from build123d import *

# Parameters (mm, degrees)
SKETCH1_W                        = 60
SKETCH1_H                        = 65
BOSS_EXTRUDE2_DEPTH              = 3
BOSS_EXTRUDE4_DEPTH              = 150
CUT_EXTRUDE2_DEPTH               = 150
FILLET1_R                        = 10
SHELL1_T                         = -5
M10X1_25_TAPPED_HOLE1_AT_2_COUNT = 2
M10X1_25_TAPPED_HOLE1_AT_2_PITCH = 42.5


with BuildPart() as part:
    # Sketch1 → Boss-Extrude2 (new body)
    with BuildSketch(Plane(origin=(0, 0, 0), x_dir=(1, 0, 0), z_dir=(0, 1, 0))):
        with Locations((30, 32.5)):
            Rectangle(SKETCH1_W, SKETCH1_H)
    extrude(amount=BOSS_EXTRUDE2_DEPTH)

    # Sketch3 → Boss-Extrude4 (add)
    with BuildSketch(Plane(origin=(0, 3, 0), x_dir=(1, 0, 0), z_dir=(0, 1, 0))):
        Polygon((0, 0), (60, 0), (33.5, 60.392887062), (26.5, 60.392887062), align=None)
    extrude(amount=BOSS_EXTRUDE4_DEPTH)

    # Sketch5 → Cut-Extrude2 (cut)
    with BuildSketch(Plane.ZY):
        Polygon((-60.392887062, 3), (-5.391813619, 150.489864796), (0, 153), (0, 157.732510012), (-60.392887062, 157.732510012), align=None)
    extrude(amount=-CUT_EXTRUDE2_DEPTH, mode=Mode.SUBTRACT)

    # Fillet1
    fillet1_edges = [part.edges().sort_by_distance(p)[0] for p in [
        (0, 1.5, -65),
        (60, 1.5, -65),
    ]]
    fillet(fillet1_edges, radius=FILLET1_R)

    # Shell1
    shell1_openings = [part.faces().sort_by_distance(p)[0] for p in [
        (30, 52, 0),
    ]]
    offset(amount=SHELL1_T, openings=shell1_openings)

    # Sketch7 → M10x1.25 Tapped Hole1 (revolve, cut)
    with BuildSketch(Plane(origin=(51.25, 3, -43.980915379), x_dir=(0, 0, 1), z_dir=(1, 0, 0))):
        Polygon((0, 0), (0, 3), (4.4, 3), (4.4, 0.625), (5.025, 0), align=None)
    m10x1_25_tapped_hole1 = revolve(axis=Axis((51.25, 9.35, -43.980915379), (0, -1, 0)), mode=Mode.SUBTRACT)

    # M10x1.25 Tapped Hole1 at 2: M10x1.25 Tapped Hole1 ×2
    with Locations(*[(-i * M10X1_25_TAPPED_HOLE1_AT_2_PITCH, 0, 0) for i in range(1, M10X1_25_TAPPED_HOLE1_AT_2_COUNT)]):
        add(m10x1_25_tapped_hole1, mode=Mode.SUBTRACT)


solid = part.part
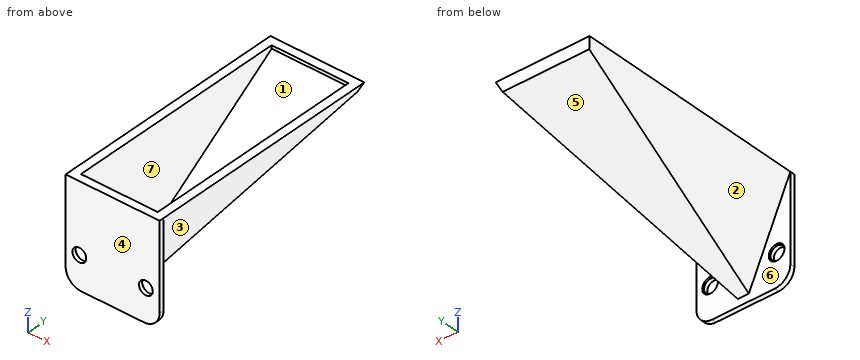
Check sheet for the modelled part. Datum: model origin and axes. Units: mm. Face numbers are marked on the shaded views. A direction names the side the tool comes from. Give positions to 0.01 mm unless a question says otherwise; leave off trailing zeros. Order: outer loops, then holes, each group sorted by start corner. A loop starts at its lowest first (then second) coordinate and runs counter-clockwise, first axis right, second up. Notation, with made-up numbers: (78.5, 25.25) - (137.5, 25.25) arc R32 ccw to (137.5, 59.25) - close; hole circle Ø9 at (56.25, 47). An arc over 180 degrees is marked (long way). Answer as CSV lines item,"result".
1. Section check A-A (z = -13). Record the boundary of the cut face in (x, y).
Result sheet:
outline,"(0, 0) - (60, 0) - (60, 3) - (54.3, 3) - (54.3, 130.09) - (5.7, 130.09) - (5.7, 3) - (0, 3) - close; hole (11.16, 5) - (48.84, 5) - (48.84, 115.78) - (11.16, 115.78) - close"
2. Mould release check, pull along X, two halves, no side actions. Record for the marked faces 1, 2, 3 and 4: released by +X, released by -X, zero draft, split by the parting line, or undercut.
Result sheet:
face 1,"undercut"
face 2,"released by -X"
face 3,"released by +X"
face 4,"zero draft"
3. Tool access check on the marked faces 5, 6 and 7. Record the directions out of +Z, -Z, +X, -X, +Y, -Y that give a thin tool (end or side, any length) a straight path to the whole face; none if there is none.
Result sheet:
face 5,"-Z, +X, -X, +Y"
face 6,"-Z, +Y"
face 7,"+Z"
4. Section check C-C (y = 88.5). Record the boundary of the cut face in (x, z).
Result sheet:
outline,"(0, 0) - (12.51, -28.51) - (47.49, -28.51) - (60, 0) - (54.54, 0) - (44.37, -23.17) - (15.63, -23.17) - (5.46, 0) - close"
5. Section check D-D (z = -25.5). Record the boundary of the cut face in (x, y).
Result sheet:
outline,"(0, 0) - (60, 0) - (60, 3) - (48.81, 3) - (48.81, 96.57) - (11.19, 96.57) - (11.19, 3) - (0, 3) - close; hole (16.65, 5) - (43.35, 5) - (43.35, 82.26) - (16.65, 82.26) - close"
6. Go/stop test with flat-tipped pins: P1, Ø4, axis at x = 35, z = -14, coming from the -Y side; P2, Ø1.5, axis at x = 30.5, y = 104.5, coming from the +Z side; P3, Ø1, axis at y = 69, z = -30.5, coming from the -X side; P4, Ø4, axis at y = 90.5, z = -22, coming from the -X side. Record where each tip stops, or that it passes through.
Result sheet:
P1,"y = 0"
P2,"z = -16.93"
P3,"x = 13.16"
P4,"x = 8.78"
7. Scan lines: probe 1 along Y at (x, z) = (4, -35.5); probe 2 along Z at (x, y) = (8, 1); probe 3 along X at (y, z) = (40, -11). Record each from-to range of solid material in increasing order. Write a range as from..to.
Result sheet:
probe 1,"0..3"
probe 2,"-64.8..-48.32, -39.65..0"
probe 3,"4.83..10.29, 49.71..55.17"
8. Section check B-B (y = 71). Record the boundary of the cut face in (x, z), then the cut area to 3 significant figures.
Result sheet:
outline,"(0, 0) - (15.37, -35.03) - (44.63, -35.03) - (60, 0) - (54.54, 0) - (41.51, -29.7) - (18.49, -29.7) - (5.46, 0) - close"
area,"493 mm²"
